Work out the finished part from the listing and answer in its coordinate system (mm). A direction names the side the tool comes from. Coordinates: 2 decimals unless noted, no trailing zeros. Order: outer loops, then holes, each group sorted by start corner. A loop starts at its lowest first (then second) coordinate and runs counter-clockwise, first axis right, second up.
1. The part is cut by section B-B, the plane x = -10.5. Give the vertices of the cut face in (y, z) (3 decimals), then the cut area to 4 significant figures.
2. The part is cut by section C-C, the plane z = -27.5. Give the vertices of the cut face in (x, y) (3 decimals), then the cut area to 3 significant figures.
3. Flat-ended cylindrical pins translate along their axes: pin 1 Ø1.1 at (x, z) = (10.5, -27.5) entering from +Y; pin 2 Ø1.5 at (y, z) = (-0.5, 10) entering from +X; pin 3 Ø3 at (x, z) = (0, 0) entering from -Y; pin 4 Ø1.5 at (x, y) = (3.5, -0.5) entering from -Z. Find the tip coordinate at first contact, or state that the pin passes through.
4. Find the intervals of material crossed by probe 1 along Z at (x, y) = (0, -1.1); probe 2 along X at (y, z) = (-0.65, -5); probe 3 along Z at (x, y) = (10.5, -0.15) (3 decimals), in increasing order.
5. The part is cut by section A-A, the plane z = -5. Give the vertices of the cut face in (x, y).
6. Determine the mould class of faces 1 (the cylindrical face through (-4.715, 0.021, 29.699)), 2 (the flat face through (-5, 0, 15)), 3 (the cylindrical face through (10.42, -0.02, -28.12)) for opening direction Z: +Z half, -Z half, draft (parallel to the pull), parting line (faces both ways), or undercut.
7. A tool of negligible diameter and unlimited length cuts with its end or side. For faces 4 (the cylindrical face through (-8.215, -0.021, -10.301)), 5 (the flat face through (5, 0, 15)), 6 (the flat face through (-9, 0, 0)), 7 (the flat face through (11, 0, -30)), from which of +Z, -Z, +X, -X, +Y, -Y can it reach the whole face along a straight path? Write none if from no direction.
8. The part is cut by section D-D, the plane y = -0.3. Give the vertices of the cut face in (x, z) (3 decimals).
```python
from build123d import *

# Parameters (mm, degrees)
SKETCH1_R           = 1.25
SKETCH1_R_2         = 0.625
BOSS_EXTRUDE1_DEPTH = 1.5
FILLET1_R           = 1


with BuildPart() as part:
    # Sketch1 → Boss-Extrude1 (new body, symmetric)
    with BuildSketch(Plane(origin=(0, 0, 0), x_dir=(1, 0, 0), z_dir=(0, 1, 0))):
        Polygon((-5, 0), (-5, -30), (5, -30), (5, 0), (12.5, 0), (12.5, 30), (8.5, 30), (8.5, 10), (-8.5, 10), (-8.5, 30), (-12.5, 30), (-12.5, 0), align=None)
        Circle(SKETCH1_R, mode=Mode.SUBTRACT)
        with Locations((0, -25.5)):
            Circle(SKETCH1_R, mode=Mode.SUBTRACT)
        with Locations((0, -12.75)):
            Circle(SKETCH1_R, mode=Mode.SUBTRACT)
        with Locations((-6.5, 5)):
            Circle(SKETCH1_R, mode=Mode.SUBTRACT)
        with Locations((6.5, 5)):
            Circle(SKETCH1_R, mode=Mode.SUBTRACT)
        with Locations((-10.5, 27.5)):
            Circle(SKETCH1_R_2, mode=Mode.SUBTRACT)
        with Locations((10.5, 27.5)):
            Circle(SKETCH1_R_2, mode=Mode.SUBTRACT)
    extrude(amount=BOSS_EXTRUDE1_DEPTH, both=True)

    # Fillet1
    fillet1_edges = [part.edges().sort_by_distance(p)[0] for p in [
        (8.5, 0, -10),
        (5, 0, 0),
        (5, 0, 30),
        (-5, 0, 30),
        (-5, 0, 0),
        (-8.5, 0, -10),
    ]]
    fillet(fillet1_edges, radius=FILLET1_R)


solid = part.part
```
Geometry says:
1. outline: (-1.5, -30) - (1.5, -30) - (1.5, -28.125) - (-1.5, -28.125) - close; (-1.5, -26.875) - (1.5, -26.875) - (1.5, 0) - (-1.5, 0) - close
1. area: 86.25 mm2
2. outline: (-12.5, -1.5) - (-11.125, -1.5) - (-11.125, 1.5) - (-12.5, 1.5) - close; (-9.875, -1.5) - (-8.5, -1.5) - (-8.5, 1.5) - (-9.875, 1.5) - close; (8.5, -1.5) - (9.875, -1.5) - (9.875, 1.5) - (8.5, 1.5) - close; (11.125, -1.5) - (12.5, -1.5) - (12.5, 1.5) - (11.125, 1.5) - close
2. area: 16.5 mm2
3. pin 1: passes through
3. pin 2: stops at x = 5
3. pin 3: stops at y = -1.5
3. pin 4: stops at z = -10
4. probe 1: z = -10 to -1.25, 1.25 to 11.5, 14 to 24.25, 26.75 to 30
4. probe 2: x = -12.5 to -7.75, -5.25 to 5.25, 7.75 to 12.5
4. probe 3: z = -30 to -28.125, -26.875 to 0
5. outline: (-12.5, -1.5) - (-7.75, -1.5) - (-7.75, 1.5) - (-12.5, 1.5) - close; (-5.25, -1.5) - (5.25, -1.5) - (5.25, 1.5) - (-5.25, 1.5) - close; (7.75, -1.5) - (12.5, -1.5) - (12.5, 1.5) - (7.75, 1.5) - close
6. face 1: +Z half
6. face 2: draft
6. face 3: undercut
7. face 4: -Z, +Y, -Y
7. face 5: +Z, +X, +Y, -Y
7. face 6: +Z, -X, +Y, -Y
7. face 7: -Z, +X, -X, +Y, -Y
8. outline: (-12.5, -30) - (-8.5, -30) - (-8.5, -11) arc R1 cw to (-7.5, -10) - (7.5, -10) arc R1 cw to (8.5, -11) - (8.5, -30) - (12.5, -30) - (12.5, 0) - (6, 0) arc R1 cw to (5, 1) - (5, 29) arc R1 ccw to (4, 30) - (-4, 30) arc R1 ccw to (-5, 29) - (-5, 1) arc R1 cw to (-6, 0) - (-12.5, 0) - close; hole circle Ø1.25 at (-10.5, -27.5); hole circle Ø2.5 at (-6.5, -5); hole circle Ø2.5 at (0, 0); hole circle Ø2.5 at (0, 12.75); hole circle Ø2.5 at (0, 25.5); hole circle Ø2.5 at (6.5, -5); hole circle Ø1.25 at (10.5, -27.5)
